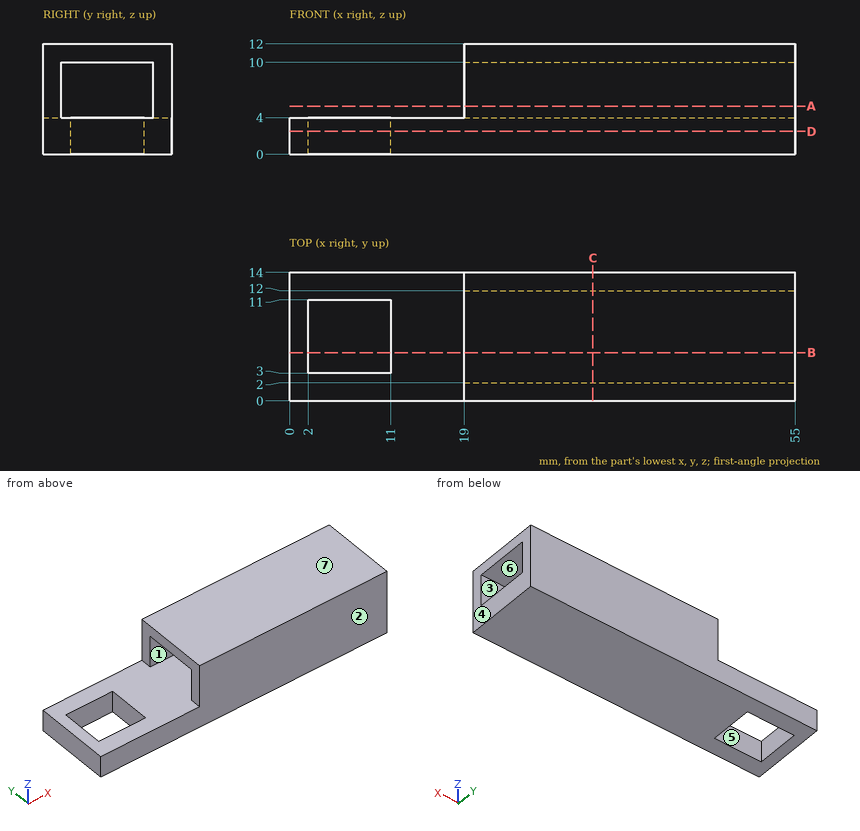
Verification items for this drawing (mm, ordinates from the low corner). A direction names the side the tool comes from. Give positions to 0.01 mm unless a question says otherwise; leave off trailing zeros. Loops run counter-clockwise (first coordinate to the right, second up) from the corner with the lowest first, then second, coordinate; pieces in that order, holes last.
1. Cross-section at A-A on z = 5.25. Record the cut outline in (x, y), and give its area (3 significant figures).
Derived:
outline: (19, 0) - (55, 0) - (55, 2) - (19, 2) - close; (19, 12) - (55, 12) - (55, 14) - (19, 14) - close
area: 144 mm2
2. Cross-section at C-C on x = 33. Record the cut outline in (y, z).
Derived:
outline: (0, 0) - (14, 0) - (14, 12) - (0, 12) - close; hole (2, 4) - (12, 4) - (12, 10) - (2, 10) - close
3. Cross-section at B-B on y = 5.25. Record the cut outline in (x, z).
Derived:
outline: (0, 0) - (2, 0) - (2, 4) - (0, 4) - close; (11, 0) - (55, 0) - (55, 4) - (11, 4) - close; (19, 10) - (55, 10) - (55, 12) - (19, 12) - close
4. Tool access check on the marked faces 5, 6 and 7. Record the directions out of +Z, -Z, +X, -X, +Y, -Y that give a thin tool (end or side, any length) a straight path to the whole face; none if there is none.
Derived:
face 5: +Z, -Z
face 6: +X, -X
face 7: +Z, +X, -X, +Y, -Y
5. Release check for a two-part mould opening along Y. For the marked faces 1, 2, 3 and 4 record: +Y half, -Y half, draft (parallel to the pull), parting line (faces both ways), or undercut.
Derived:
face 1: undercut
face 2: -Y half
face 3: undercut
face 4: draft
6. Cross-section at D-D on z = 2.5. Record the cut outline in (x, y), and give its area (3 significant figures).
Derived:
outline: (0, 0) - (55, 0) - (55, 14) - (0, 14) - close; hole (2, 3) - (11, 3) - (11, 11) - (2, 11) - close
area: 698 mm2
7. Material ranges on probe 1 along Z at (x, y) = (34, 2.5); probe 2 along Y at (x, z) = (52, 5.25); probe 3 along X at (y, z) = (3.5, 2), recorded low to high.
Derived:
probe 1: z = 0 to 4, 10 to 12
probe 2: y = 0 to 2, 12 to 14
probe 3: x = 0 to 2, 11 to 55
8. Go/stop test with flat-tipped pins: P1, Ø7, axis at x = 14.5, y = 5.5, coming from the +Z side; P2, Ø4, axis at y = 8.5, z = 9, coming from the -X side; P3, Ø2, axis at x = 16, z = 6, coming from the -Y side. Record where each tip stops, or that it passes through.
Derived:
P1: stops at z = 4
P2: stops at x = 19
P3: passes through
